The listing builds one solid part. Answer for the finished solid, in the listing's coordinates (mm). Face numbers are marked on the shaded views. A direction names the side the tool comes from. Round coordinates to 2 decimals unless told otherwise and drop trailing zeros. Order: outer loops, then holes, each group sorted by start corner. A loop starts at its lowest first (then second) coordinate and runs counter-clockwise, first axis right, second up. Notation, with made-up numbers: (26, 79.5) - (67, 79.5) arc R15 ccw to (67, 89.5) - close; hole circle Ø8 at (53.5, -5). An arc over 180 degrees is marked (long way). Write item = value, one per line.
from build123d import *

# Parameters (mm, degrees)
FILLET1_R           = 1
FILLET2_R           = 2
SKETCH2_R           = 0.375
BOSS_EXTRUDE1_DEPTH = 7
CIRPATTERN1_COUNT   = 14
CIRPATTERN1_ANGLE   = 312


with BuildPart() as part:
    # Sketch1 → Revolve1 (revolve)
    with BuildSketch(Plane(origin=(0, 0, 0), x_dir=(0, 0, -1), z_dir=(1, 0, 0)), mode=Mode.PRIVATE) as revolve1_sk:
        Polygon((0, 0), (0, 16.25), (90, 16.25), (96, 13), (99, 13), (99, 3), (111, 3), (111, 0), align=None)
    revolve(revolve1_sk.sketch.rotate(Axis((0, 0, -111), (0, 0, -1)), 90), axis=Axis((0, 0, -111), (0, 0, -1)))

    # Fillet1
    fillet1_edges = [part.edges().sort_by_distance(p)[0] for p in [
        (-13, 0, -99),
        (-16.25, 0, 0),
    ]]
    fillet(fillet1_edges, radius=FILLET1_R)

    # Fillet2
    fillet2_edges = [part.edges().sort_by_distance(p)[0] for p in [
        (-3, 0, -111),
        (-3, 0, -99),
        (-13, 0, -96),
        (-16.25, 0, -90),
    ]]
    fillet(fillet2_edges, radius=FILLET2_R)

    # Sketch2 → Boss-Extrude1 (add)
    with BuildSketch(Plane(origin=(0, 0, -99), x_dir=(-1, 0, 0), z_dir=(0, 0, -1))):
        with Locations(Location((3.863998109, -8.678681848, 0), (0, 0, 180))):
            Circle(SKETCH2_R)
    boss_extrude1 = extrude(amount=BOSS_EXTRUDE1_DEPTH)

    # CirPattern1: Boss-Extrude1 ×14 about axis
    cirpattern1_axis = Axis((0, 0, 0), (0, 0, -1))
    for i in range(1, CIRPATTERN1_COUNT):
        add(boss_extrude1.rotate(cirpattern1_axis, i * CIRPATTERN1_ANGLE / (CIRPATTERN1_COUNT - 1)))


solid = part.part
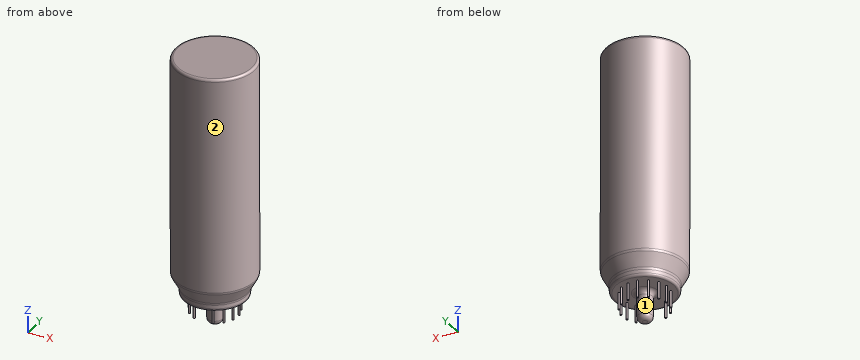
Q1. Section A-A on z = -94 is taken. Determine the outline of the cut face in (x, y), then the cut area to 3 significant figures.
Model answer:
outline = circle Ø28.17 at (0, 0)
area = 623 mm^2
Q2. Find the intervals of material crossed by line 1 (Z direction, x = 5.5, y = 2); line 2 (Y direction, x = -12.5, z = -44); line 3 (Y direction, x = 7.5, z = -71), in increasing order. Write a range as from..to.
Model answer:
line_1 = -99..0
line_2 = -10.38..10.38
line_3 = -14.42..14.42
Q3. For the marked faces 1 and 2, determine the directions among +Z, -Z, +X, -X, +Y, -Y from which every point of the face is accessible in a straight line to the end or side of a thin tool.
Model answer:
face_1 = -Z
face_2 = +Z, -Z
Q4. Flat-ended cylindrical pins translate along their axes: P1, Ø0.6, axis at x = 7, y = -6.5, coming from the -Z side; P2, Ø8, axis at x = -8.5, z = -37.5, coming from the +Y side; P3, Ø1, axis at y = 6, z = -86, coming from the -X side. Find the tip coordinate at first contact, or state that the pin passes through.
Model answer:
P1 = -106
P2 = 15.61
P3 = -15.29
Q5. Section B-B on z = -53 is taken. Determine the outline of the cut face in (x, y).
Model answer:
outline = circle Ø32.5 at (0, 0)
